```python
from build123d import *

# Parameters (mm, degrees)
SKETCH1_R           = 2.5
BOSS_EXTRUDE2_DEPTH = 4
FILLET1_R           = 5
SKETCH2_R           = 5
SKETCH2_R_2         = 2.5
SKETCH2_R_3         = 2.410622894
BOSS_EXTRUDE3_DEPTH = 7
FILLET2_R           = 2.5
SKETCH3_R           = 2.5
CUT_EXTRUDE1_DEPTH  = 80.510690177


with BuildPart() as part:
    # Sketch1 → Boss-Extrude2 (new body)
    with BuildSketch(Plane(origin=(0, 0, 0), x_dir=(1, 0, 0), z_dir=(0, 1, 0))):
        Polygon((-2.997842525, 1.627546264), (-2.997842525, -22.606832334), (7.911575214, -43.612950039), (31.557320362, -43.612950039), (55.203065509, -43.612950039), (66.112483248, -22.606832334), (66.112483248, 1.627546264), (38.728999177, 28.237162663), (24.385641546, 28.237162663), align=None)
        with Locations(Location((55.490124242, -20.289109104, 0), (0, 0, 270))):
            Circle(SKETCH1_R, mode=Mode.SUBTRACT)
        with Locations(Location((31.557320362, 19.710890896, 0), (0, 0, 270))):
            Circle(SKETCH1_R, mode=Mode.SUBTRACT)
        with Locations(Location((7.624516482, -20.289109104, 0), (0, 0, 270))):
            Circle(SKETCH1_R, mode=Mode.SUBTRACT)
    extrude(amount=BOSS_EXTRUDE2_DEPTH)

    # Fillet1
    fillet1_edges = [part.edges().sort_by_distance(p)[0] for p in [
        (24.385641546, 2, -28.237162663),
        (38.728999177, 2, -28.237162663),
        (66.112483248, 2, -1.627546264),
        (66.112483248, 2, 22.606832334),
        (55.203065509, 2, 43.612950039),
        (7.911575214, 2, 43.612950039),
        (-2.997842525, 2, 22.606832334),
        (-2.997842525, 2, -1.627546264),
    ]]
    fillet(fillet1_edges, radius=FILLET1_R)

    # Sketch2 → Boss-Extrude3 (add)
    # profile 1 of 3: a face of its own
    with BuildSketch(Plane(origin=(0, 4, 0), x_dir=(1, 0, 0), z_dir=(0, 1, 0))):
        with Locations(Location((31.557320362, 19.710890896, 0), (0, 0, 270))):
            Circle(SKETCH2_R)
        with Locations(Location((31.557320362, 19.710890896, 0), (0, 0, 270))):
            Circle(SKETCH2_R_2, mode=Mode.SUBTRACT)
    # profile 2 of 3: a face of its own
    with BuildSketch(Plane(origin=(0, 4, 0), x_dir=(1, 0, 0), z_dir=(0, 1, 0))):
        with Locations(Location((55.490124242, -20.289109104, 0), (0, 0, 270))):
            Circle(SKETCH2_R)
        with Locations(Location((55.490124242, -20.289109104, 0), (0, 0, 270))):
            Circle(SKETCH2_R_2, mode=Mode.SUBTRACT)
    # profile 3 of 3: a face of its own
    with BuildSketch(Plane(origin=(0, 4, 0), x_dir=(1, 0, 0), z_dir=(0, 1, 0))):
        with Locations(Location((7.624516482, -20.289109104, 0), (0, 0, 270))):
            Circle(SKETCH2_R)
        with Locations(Location((7.624516482, -20.289109104, 0), (0, 0, 270))):
            Circle(SKETCH2_R_3, mode=Mode.SUBTRACT)
    extrude(amount=BOSS_EXTRUDE3_DEPTH)

    # Fillet2
    fillet2_edges = [part.edges().sort_by_distance(p)[0] for p in [
        (55.490124242, 4, 15.289109104),
        (7.624516482, 4, 15.289109104),
        (31.557320362, 4, -24.710890896),
    ]]
    fillet(fillet2_edges, radius=FILLET2_R)

    # Sketch3 → Cut-Extrude1 (cut, through all)
    with BuildSketch(Plane(origin=(0, 4, 0), x_dir=(1, 0, 0), z_dir=(0, 1, 0))):
        with Locations(Location((39.057320362, -34.521990264, 0), (0, 0, 270))):
            Circle(SKETCH3_R)
        with Locations(Location((24.057320362, -34.521990264, 0), (0, 0, 270))):
            Circle(SKETCH3_R)
    extrude(amount=-CUT_EXTRUDE1_DEPTH, mode=Mode.SUBTRACT)


solid = part.part
```
For this review, take the finished solid that the model builds, in its own axes (mm). A direction names the side the tool comes from. Round coordinates to 2 decimals unless told otherwise and drop trailing zeros. Loops run counter-clockwise (first coordinate to the right, second up) from the corner with the lowest first, then second, coordinate; pieces in that order, holes last.
Q1. Mouldability with a two-part tool opening along X and no side actions: class faces 4 (the face through (30.6, 5.4, -17.4)), 5 (the face through (26.676, 8.718, -20.795)), 6 (the face through (59.706, 8.718, 22.977)), 7 (the face through (8.32, 2.028, 42.866)) as +X half, -X half, draft (parallel to the pull), parting line (faces both ways), or undercut.
Result sheet:
face 4: undercut
face 5: parting line
face 6: undercut
face 7: -X half
Q2. Add section A-A on y = 1.75. Write out the cut boundary in (x, z), plus the area to 3 significant figures.
Result sheet:
outline: (-3, 0.49) arc R5 ccw to (-1.48, -3.1) - (22.93, -26.82) arc R5 ccw to (26.41, -28.24) - (36.7, -28.24) arc R5 ccw to (40.18, -26.82) - (64.6, -3.1) arc R5 ccw to (66.11, 0.49) - (66.11, 21.39) arc R5 ccw to (65.55, 23.69) - (56.6, 40.92) arc R5 ccw to (52.17, 43.61) - (10.95, 43.61) arc R5 ccw to (6.51, 40.92) - (-2.44, 23.69) arc R5 ccw to (-3, 21.39) - close; hole circle Ø5 at (7.62, 20.29); hole circle Ø5 at (24.06, 34.52); hole circle Ø5 at (31.56, -19.71); hole circle Ø5 at (39.06, 34.52); hole circle Ø5 at (55.49, 20.29)
area: 3,900 mm2
Q3. Insertion check: pin 1 Ø2.5 at (x, z) = (7.5, 19.5) entering from -Y; pin 2 Ø1 at (x, y) = (27, 8) entering from -Z; pin 3 Ø1.5 at (y, z) = (4, -12) entering from -X; pin 4 Ø1 at (x, y) = (8.5, 4) entering from +Z. Each pin has a flat end and moves straight along its axis. Give the tip position at first contact, or say it passes through.
Result sheet:
pin 1: passes through
pin 2: stops at z = -22.63
pin 3: stops at x = 6.9
pin 4: stops at z = 43.22
Q4. To check wall thickness, follow line 1 along X through (y, z) = (3, 21.5); line 2 along Y through (x, z) = (52, -4); line 3 along X through (y, z) = (8.5, -17.5). State the ranges of each line that lie inside material, in increasing order.
Result sheet:
line 1: x = -3 to 5.44, 9.81 to 53.3, 57.68 to 66.11
line 2: y = 0 to 4
line 3: x = 27.07 to 30.39, 32.72 to 36.04
Q5. Add section B-B on y = 5.5. Write out the cut boundary in (x, z).
Result sheet:
outline: circle Ø10.42 at (7.62, 20.29); circle Ø10.42 at (31.56, -19.71); circle Ø10.42 at (55.49, 20.29); hole circle Ø4.82 at (7.62, 20.29); hole circle Ø5 at (31.56, -19.71); hole circle Ø5 at (55.49, 20.29)
Q6. Machinability: for faces 1 (the face through (2.743, 8.718, 19.205)), 2 (the face through (66.112, 2, 11)), 3 (the face through (6.67, 1.97, 22.6)), which of the approach directions +Z, -Z, +X, -X, +Y, -Y give a long, thin tool a straight path to every point of the face, cutting with its end or side? Answer none if there is none.
Result sheet:
face 1: +Y
face 2: +Z, -Z, +X, +Y, -Y
face 3: -Y
Q7. Add section D-D on z = -5. Write out the cut boundary in (x, y), plus the area to 3 significant figures.
Result sheet:
outline: (0.47, 0) - (62.64, 0) - (62.64, 4) - (0.47, 4) - close
area: 249 mm2
Q8. Add section C-C on z = 8. Write out the cut boundary in (x, y).
Result sheet:
outline: (-3, 0) - (66.11, 0) - (66.11, 4) - (-3, 4) - close
